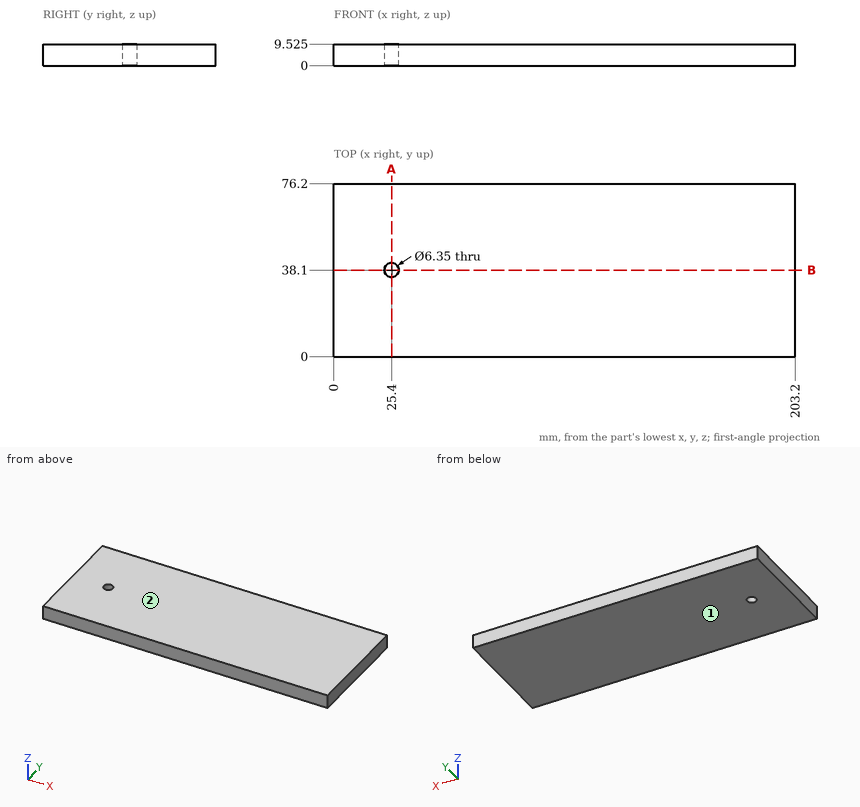
Source: three-view drawing plus pictorial views. Frame: mm from the lowest corner of the part. Coordinates: 2 decimals unless noted, no trailing zeros. Order: outer loops, then holes, each group sorted by start corner. A loop starts at its lowest first (then second) coordinate and runs counter-clockwise, first axis right, second up. Notation, with made-up numbers: M 17.5,46.5 L 23.5,46.5 A20 ccw 23.5,82.5 Z; hole C 51,50 d6. An arc over 180 degrees is marked long. Answer in a Markdown table with one row per item.
(1) Contact query for flat-ended pins moving along their axis: pin 1 Ø5 at (y, z) = (57, 1.5) entering from -X; pin 2 Ø4 at (x, y) = (25.4, 38.1) entering from -Z. Output: stop coordinate, or through.
Numbers:
| item | result |
|---|---|
| pin 1 | stops at x = 0 |
| pin 2 | passes through |
(2) Section query B-B, the plane y = 38.1. Output: boundary loops of the cut face in (x, z) (3 decimals), plus the area to 4 significant figures.
Numbers:
| item | result |
|---|---|
| outline | M 0,0 L 22.225,0 L 22.225,9.525 L 0,9.525 Z; M 28.575,0 L 203.2,0 L 203.2,9.525 L 28.575,9.525 Z |
| area | 1,875 mm^2 |
(3) Draft query along Z for the marked faces 1 and 2. Return one class per face: pulls with the +Z half, pulls with the -Z half, needs draft (parallel to the pull), parting line crosses it, or undercut.
Numbers:
| item | result |
|---|---|
| face 1 | pulls with the -Z half |
| face 2 | pulls with the +Z half |
(4) Section query A-A, the plane x = 25.4. Output: boundary loops of the cut face in (y, z) (3 decimals), plus the area to 3 significant figures.
Numbers:
| item | result |
|---|---|
| outline | M 0,0 L 34.925,0 L 34.925,9.525 L 0,9.525 Z; M 41.275,0 L 76.2,0 L 76.2,9.525 L 41.275,9.525 Z |
| area | 665 mm^2 |
(5) Material intervals for line 1 (X direction, y = 38, z = 5.25); line 2 (Y direction, x = 25.4, z = 2.75) (3 decimals); line 3 (X direction, y = 40.5, z = 9), sorted ascending. Write a range as [from, to].
Numbers:
| item | result |
|---|---|
| line 1 | x = [0, 22.23], [28.57, 203.2] |
| line 2 | y = [0, 34.925], [41.275, 76.2] |
| line 3 | x = [0, 23.32], [27.48, 203.2] |
